Geometry check sheet. Reference: the model listing, model coordinates, mm. A direction names the side the tool comes from. Round coordinates to 2 decimals unless told otherwise and drop trailing zeros. Order: outer loops, then holes, each group sorted by start corner. A loop starts at its lowest first (then second) coordinate and runs counter-clockwise, first axis right, second up.
(1) Cross-section at A-A on z = 22.5. Enter the section's corners in (x, y).
(2) Gauge pin test, flat ends, axial feed: P1, Ø10, axis at y = -10, z = -50, coming from the +X side; P2, Ø6, axis at x = 11.5, z = -35.5, coming from the +Y side; P3, Ø4, axis at x = -4.5, z = -6.5, coming from the -Y side. Record the tip position at first contact, or that the pin passes through.
(3) Thickness scan on L1, parallel to Z at x = 11, y = 9; L2, parallel to Y at x = -7.5, z = 132.5; L3, parallel to Y at x = 2, z = -191.5. Record the ranges inside material, lowest first.
(4) Set-up check for faces 3 (the face through (-2.17, -9.76, 236.2)), 4 (the face through (0, 0, 250)): record each of +Z, -Z, +X, -X, +Y, -Y from which the full face is reachable in a straight line by a thin tool's end or side.
(5) Draft check along X on faces 1 (the face through (0, 0, -250)), 2 (the face through (-4.336, -19.524, 1.301)). Enter one of: pulls with the +X half, pulls with the -X half, needs draft (parallel to the pull), parting line crosses it, or undercut.
from build123d import *


# Not quite as in the source:
# - a feature names something its author has since deleted; it is built from what else it names


with BuildPart() as f1:
    # F0 (on Front) → F1 (revolve)
    with BuildSketch(Plane.XZ):
        with BuildLine():
            Line((0, 250), (0, 0))
            Line((0, 0), (0, -250))
            Line((0, -250), (15, -250))
            add(Edge.make_bspline(
                [(15, -250), (13.4045789018, -193.5875862837), (17.3846632242, -147.1532583237), (20, -92.9462272166)],
                knots=[0, 0, 0, 0, 157.1333432009, 157.1333432009, 157.1333432009, 157.1333432009], degree=3))
            Line((20, -92.9462272166), (20, 0))
            Line((20, 0), (20, 92.9462272166))
            add(Edge.make_bspline(
                [(15, 222), (16.6666666667, 181.3154090722), (18.3333333333, 133.6308181444), (20, 92.9462272166)],
                knots=[0, 0, 0, 0, 129.1505953127, 129.1505953127, 129.1505953127, 129.1505953127], degree=3))
            Line((15, 222), (10, 222))
            Line((10, 222), (10, 250))
            Line((10, 250), (0, 250))
        make_face()
    revolve(axis=Axis((0, 0, 125), (0, 0, 1)))


solid = f1.part
Found:
1. outline: circle Ø40 at (0, 0)
2. P1: stops at x = 19.36
2. P2: stops at y = 18.1
2. P3: stops at y = -19.84
3. L1: z = -250 to 222
3. L2: y = -16.85 to 16.85
3. L3: y = -15.01 to 15.01
4. face 3: +Z
4. face 4: +Z, +X, -X, +Y, -Y
5. face 1: needs draft
5. face 2: parting line crosses it
